Can you work these out from the model? Positions are in its coordinate system, mm. Give positions to 0.01 mm unless a question says otherwise; leave off trailing zeros. Loops run counter-clockwise (first coordinate to the right, second up) from the corner with the lowest first, then second, coordinate; pieces in that order, holes last. Notation, with made-up numbers: M 43.5,44 L 88.5,44 A31 ccw 88.5,81 Z; hole C 59,64.25 d2. An arc over 180 degrees is marked long. Put each result on its own line as item: value. Start each with the question number.
1) Imagine slicing it at D-D (y = -30.5). Write out the boundary of the cut face in (x, z).
2) Please list where these lines run through material, in increasing order: line 1 along Y through (x, z) = (15.4, 2.25); line 2 along Y through (x, z) = (16.5, 1.8); line 3 along Y through (x, z) = (94.5, 4.65). Write a range as from..to.
3) If we mould it in two halves opening along Y, with no side actions, what happens to faces 1 (the flat face through (53.995, 21.749, 2.465)), 2 (the cylindrical face through (10.36, -44.29, 2.46)), 3 (the cylindrical face through (16.01, 34.17, 2.46))? For each: +Y half, -Y half, draft (parallel to the pull), parting line (faces both ways), or undercut.
4) Imagine slicing it at B-B (x = 30). Write out the boundary of the cut face in (y, z).
5) For P1, Ø1.5, axis at x = 137, z = 3.5, coming from the -Y side; P2, Ø4, axis at x = 120.54, y = 0, coming from the +Z side; P3, Ø3, axis at y = 25.5, z = 3.5, coming from the -X side, each with a flat end and sliding along its axis, tell me the tip position at first contact or that it passes through.
6) Imagine slicing it at C-C (x = 56). Write out the boundary of the cut face in (y, z), then the cut area to 3 significant figures.
7) Imagine slicing it at A-A (z = 4.2). State how many separate pieces and enclosed holes the cut face has, then the cut area to 3 significant figures.
from build123d import *

# Parameters (mm, degrees)
CROQUIS1_R              = 2.25
CROQUIS1_R_2            = 2.55
CROQUIS1_R_3            = 1.5
SALIENTE_EXTRUIR1_DEPTH = 5
SALIENTE_EXTRUIR2_START = -5
CROQUIS2_R              = 2.55
CROQUIS2_R_2            = 1.5
SALIENTE_EXTRUIR2_DEPTH = 5


with BuildPart() as part:
    # Croquis1 → Saliente-Extruir1 (new body)
    with BuildSketch(Plane(origin=(0, 0, 0), x_dir=(-1, 0, 0), z_dir=(0, 0, -1))):
        with BuildLine():
            Line((-71.341040378, -16.363356968), (-70.419428585, -16.899757727))
            Line((-70.419428585, -16.899757727), (-20.270039886, -44.385636378))
            ThreePointArc((-20.270039886, -44.385636378), (-10.236419944, -44.21832916), (-5.267289487, -35.5))
            Line((-5.267289487, -35.5), (-5.267289487, 34.708239567))
            ThreePointArc((-5.267289487, 34.708239567), (-11.664110706, 44.896341112), (-23.263165727, 41.705940291))
            ThreePointArc((-23.263165727, 41.705940291), (-30.502802881, 34.357904526), (-39.225518904, 28.851526324))
            Line((-39.225518904, 28.851526324), (-69.184263586, 14.445246544))
            ThreePointArc((-69.184263586, 14.445246544), (-78.684950229, 11.125383731), (-88.685852551, 10))
            Line((-88.685852551, 10), (-120.543509993, 10))
            Line((-120.543509993, 10), (-161.221070033, 10))
            ThreePointArc((-161.221070033, 10), (-171.221070033, 0), (-161.221070033, -10))
            Line((-161.221070033, -10), (-120.543509993, -10))
            Line((-120.543509993, -10), (-93.547882821, -10.2575901))
            ThreePointArc((-93.547882821, -10.2575901), (-82.047232991, -11.865742134), (-71.341040378, -16.363356968))
        make_face()
        with Locations(Location((-30, 0, 0), (0, 0, 180))):
            Circle(CROQUIS1_R, mode=Mode.SUBTRACT)
        with Locations(Location((-15.4, -35.5, 0), (0, 0, 180))):
            Circle(CROQUIS1_R_2, mode=Mode.SUBTRACT)
        with Locations(Location((-15.317880165, 35.5, 0), (0, 0, 180))):
            Circle(CROQUIS1_R_2, mode=Mode.SUBTRACT)
        with Locations(Location((-141.14380115, 0, 0), (0, 0, 180))):
            Circle(CROQUIS1_R, mode=Mode.SUBTRACT)
        with Locations(Location((-161.221070033, 0, 0), (0, 0, 180))):
            Circle(CROQUIS1_R, mode=Mode.SUBTRACT)
        with Locations(Location((-56, 0, 0), (0, 0, 180))):
            Circle(CROQUIS1_R, mode=Mode.SUBTRACT)
        with Locations(Location((-75.6, 0, 0), (0, 0, 180))):
            Circle(CROQUIS1_R_3, mode=Mode.SUBTRACT)
        with Locations(Location((-99.210066217, 0, 0), (0, 0, 180))):
            Circle(CROQUIS1_R, mode=Mode.SUBTRACT)
        with Locations(Location((-120.543509993, 0, 0), (0, 0, 180))):
            Circle(CROQUIS1_R, mode=Mode.SUBTRACT)
    extrude(amount=-SALIENTE_EXTRUIR1_DEPTH)

    # Croquis2 → Saliente-Extruir2 (add)
    # profile 1 of 2: a face of its own
    with BuildSketch(Plane.XY.offset(5).offset(SALIENTE_EXTRUIR2_START)):
        with Locations((15.4, -35.5)):
            Circle(CROQUIS2_R)
        with Locations((15.4, -35.5)):
            Circle(CROQUIS2_R_2, mode=Mode.SUBTRACT)
    # profile 2 of 2: a face of its own
    with BuildSketch(Plane.XY.offset(5).offset(SALIENTE_EXTRUIR2_START)):
        with Locations((15.317880165, 35.5)):
            Circle(CROQUIS2_R)
        with Locations((15.317880165, 35.5)):
            Circle(CROQUIS2_R_2, mode=Mode.SUBTRACT)
    extrude(amount=SALIENTE_EXTRUIR2_DEPTH)


solid = part.part
Recorded:
1. outline: M 5.27,0 L 45.61,0 L 45.61,5 L 5.27,5 Z
2. line 1: -45.63..-37, -34..34, 37..45.58
2. line 2: -45.57..-36.52, -34.48..34.58, 36.42..45.51
2. line 3: -10.25..10
3. face 1: +Y half
3. face 2: -Y half
3. face 3: undercut
4. outline: M -39.05,0 L -2.25,0 L -2.25,5 L -39.05,5 Z; M 2.25,0 L 34.77,0 L 34.77,5 L 2.25,5 Z
5. P1: y = -10
5. P2: through
5. P3: x = 5.27
6. outline: M -24.8,0 L -2.25,0 L -2.25,5 L -24.8,5 Z; M 2.25,0 L 20.79,0 L 20.79,5 L 2.25,5 Z
6. area: 205 mm²
7. separate pieces: 1
7. enclosed holes: 9
7. area: 6,140 mm²
